Build history of the part. All positions in model axes, mm. A direction names the side the tool comes from. Round coordinates to 2 decimals unless told otherwise and drop trailing zeros. Order: outer loops, then holes, each group sorted by start corner. A loop starts at its lowest first (then second) coordinate and runs counter-clockwise, first axis right, second up. Notation, with made-up numbers: (-21, -2.5) -> (11, -2.5) arc R21 ccw to (11, 21.5) -> close; hole circle Ø1 at (17.25, 56). An arc over 180 degrees is marked (long way). Use a Markdown table: item, result. Add a question column.
Item 1: Slice it at C-C, the plane x = 15.5. Give the cut face in (y, z).
Item 2: Two-plate mould, pull along X, no slides. Class faces 1 (the face through (-5.295, 5.321, 0.986)), 2 (the face through (10.451, -4.008, 0.986)), 3 (the face through (-6.1, 6.57, 0.99)): released by +X, released by -X, zero draft, split by the parting line, or undercut.
Item 3: Probe L1, parallel to X at y = -13.5, z = 0.3; L2, parallel to X at y = -18, z = 0.65; L3, parallel to Y at x = -9, z = 0.45. List the from-to ranges inside material, lowest first.
Item 4: Slice it at B-B, the plane y = -11.5. Give the cut face in (x, z), plus the area to 3 significant figures.
Item 5: 3-axis set-ups, long thin cutter, end or side, ignore diameter. For faces 4 (the face through (-8.195, -0.584, 0.986)), 5 (the face through (1.4, -1, 0)), 6 (the face through (-1.2, 8.7, 1)): which of +Z, -Z, +X, -X, +Y, -Y reach the whole face in a straight line?
Item 6: Slice it at A-A, the plane z = 1.55. State how many separate pieces and enclosed holes the cut face has, plus the area to 3 significant figures.
from build123d import *

# Parameters (mm, degrees)
F1_DEPTH = 2


with BuildPart() as f1:
    # F0 (on Top) → F1 (new body)
    with BuildSketch(Plane.XY):
        Polygon((16.885106, -21.930141), (3.835107, 14.423427), (-16.31955, -1.512813), (0.15961, 0.370519), align=None)
        with BuildLine():
            ThreePointArc((-4.606246, 4.476535), (-4.614025, 4.49657), (-4.62165, 4.516664))
            Line((-4.62165, 4.516664), (-5.270834, 4.857064))
            Line((-5.270834, 4.857064), (-5.320121, 5.797519))
            Line((-5.320121, 5.797519), (-4.710075, 6.203913))
            ThreePointArc((-4.710075, 6.203913), (-4.704592, 6.224693), (-4.69895, 6.245431))
            Line((-4.69895, 6.245431), (-5.024069, 6.902401))
            Line((-5.024069, 6.902401), (-4.511157, 7.692216))
            Line((-4.511157, 7.692216), (-3.778747, 7.662419))
            ThreePointArc((-3.778747, 7.662419), (-3.762097, 7.676009), (-3.745343, 7.68947))
            Line((-3.745343, 7.68947), (-3.622212, 8.41207))
            Line((-3.622212, 8.41207), (-2.743016, 8.749561))
            Line((-2.743016, 8.749561), (-2.167999, 8.294956))
            ThreePointArc((-2.167999, 8.294956), (-2.146541, 8.296163), (-2.125074, 8.297205))
            Line((-2.125074, 8.297205), (-1.600726, 8.809426))
            Line((-1.600726, 8.809426), (-0.691069, 8.565684))
            Line((-0.691069, 8.565684), (-0.49308, 7.859914))
            ThreePointArc((-0.49308, 7.859914), (-0.475011, 7.848278), (-0.457031, 7.836503))
            Line((-0.457031, 7.836503), (0.268252, 7.942694))
            Line((0.268252, 7.942694), (0.860912, 7.21082))
            Line((0.860912, 7.21082), (0.606246, 6.523465))
            ThreePointArc((0.606246, 6.523465), (0.614025, 6.50343), (0.62165, 6.483336))
            Line((0.62165, 6.483336), (1.270834, 6.142936))
            Line((1.270834, 6.142936), (1.320121, 5.202481))
            Line((1.320121, 5.202481), (0.710075, 4.796087))
            ThreePointArc((0.710075, 4.796087), (0.704592, 4.775307), (0.69895, 4.754569))
            Line((0.69895, 4.754569), (1.024069, 4.097599))
            Line((1.024069, 4.097599), (0.511157, 3.307784))
            Line((0.511157, 3.307784), (-0.221253, 3.337581))
            ThreePointArc((-0.221253, 3.337581), (-0.237903, 3.323991), (-0.254657, 3.31053))
            Line((-0.254657, 3.31053), (-0.377788, 2.58793))
            Line((-0.377788, 2.58793), (-1.256984, 2.250439))
            Line((-1.256984, 2.250439), (-1.832001, 2.705044))
            ThreePointArc((-1.832001, 2.705044), (-1.853459, 2.703837), (-1.874926, 2.702795))
            Line((-1.874926, 2.702795), (-2.399274, 2.190574))
            Line((-2.399274, 2.190574), (-3.308931, 2.434316))
            Line((-3.308931, 2.434316), (-3.50692, 3.140086))
            ThreePointArc((-3.50692, 3.140086), (-3.524989, 3.151722), (-3.542969, 3.163497))
            Line((-3.542969, 3.163497), (-4.268252, 3.057306))
            Line((-4.268252, 3.057306), (-4.860912, 3.78918))
            Line((-4.860912, 3.78918), (-4.606246, 4.476535))
        make_face(mode=Mode.SUBTRACT)
        with BuildLine():
            ThreePointArc((2.857031, 4.836503), (2.875011, 4.848278), (2.89308, 4.859914))
            Line((2.89308, 4.859914), (3.091069, 5.565684))
            Line((3.091069, 5.565684), (4.000726, 5.809426))
            Line((4.000726, 5.809426), (4.525074, 5.297205))
            ThreePointArc((4.525074, 5.297205), (4.546541, 5.296163), (4.567999, 5.294956))
            Line((4.567999, 5.294956), (5.143016, 5.749561))
            Line((5.143016, 5.749561), (6.022212, 5.41207))
            Line((6.022212, 5.41207), (6.145343, 4.68947))
            ThreePointArc((6.145343, 4.68947), (6.162097, 4.676009), (6.178747, 4.662419))
            Line((6.178747, 4.662419), (6.911157, 4.692216))
            Line((6.911157, 4.692216), (7.424069, 3.902401))
            Line((7.424069, 3.902401), (7.09895, 3.245431))
            ThreePointArc((7.09895, 3.245431), (7.104592, 3.224693), (7.110075, 3.203913))
            Line((7.110075, 3.203913), (7.720121, 2.797519))
            Line((7.720121, 2.797519), (7.670834, 1.857064))
            Line((7.670834, 1.857064), (7.02165, 1.516664))
            ThreePointArc((7.02165, 1.516664), (7.014025, 1.49657), (7.006246, 1.476535))
            Line((7.006246, 1.476535), (7.260912, 0.78918))
            Line((7.260912, 0.78918), (6.668252, 0.057306))
            Line((6.668252, 0.057306), (5.942969, 0.163497))
            ThreePointArc((5.942969, 0.163497), (5.924989, 0.151722), (5.90692, 0.140086))
            Line((5.90692, 0.140086), (5.708931, -0.565684))
            Line((5.708931, -0.565684), (4.799274, -0.809426))
            Line((4.799274, -0.809426), (4.274926, -0.297205))
            ThreePointArc((4.274926, -0.297205), (4.253459, -0.296163), (4.232001, -0.294956))
            Line((4.232001, -0.294956), (3.656984, -0.749561))
            Line((3.656984, -0.749561), (2.777788, -0.41207))
            Line((2.777788, -0.41207), (2.654657, 0.31053))
            ThreePointArc((2.654657, 0.31053), (2.637903, 0.323991), (2.621253, 0.337581))
            Line((2.621253, 0.337581), (1.888843, 0.307784))
            Line((1.888843, 0.307784), (1.375931, 1.097599))
            Line((1.375931, 1.097599), (1.70105, 1.754569))
            ThreePointArc((1.70105, 1.754569), (1.695408, 1.775307), (1.689925, 1.796087))
            Line((1.689925, 1.796087), (1.079879, 2.202481))
            Line((1.079879, 2.202481), (1.129166, 3.142936))
            Line((1.129166, 3.142936), (1.77835, 3.483336))
            ThreePointArc((1.77835, 3.483336), (1.785975, 3.50343), (1.793754, 3.523465))
            Line((1.793754, 3.523465), (1.539088, 4.21082))
            Line((1.539088, 4.21082), (2.131748, 4.942694))
            Line((2.131748, 4.942694), (2.857031, 4.836503))
        make_face(mode=Mode.SUBTRACT)
    extrude(amount=F1_DEPTH)


solid = f1.part
Check sheet entries:
| question | item | result |
|---|---|---|
| 1 | outline | (-20.08, 0) -> (-18.07, 0) -> (-18.07, 2) -> (-20.08, 2) -> close |
| 2 | face 1 | undercut |
| 2 | face 2 | released by +X |
| 2 | face 3 | released by -X |
| 3 | L1 | 10.56 to 13.86 |
| 3 | L2 | 13.94 to 15.47 |
| 3 | L3 | -0.68 to 4.27 |
| 4 | outline | (9.06, 0) -> (13.14, 0) -> (13.14, 2) -> (9.06, 2) -> close |
| 4 | area | 8.16 mm2 |
| 5 | face 4 | +Z, -Z, -Y |
| 5 | face 5 | -Z, +X, -X, +Y, -Y |
| 5 | face 6 | +Z, -Z |
| 6 | separate pieces | 1 |
| 6 | enclosed holes | 2 |
| 6 | area | 208 mm2 |
